```python
from build123d import *


with BuildPart() as part:
    # Sketch1 → Revolve1 (revolve)
    with BuildSketch(Plane(origin=(0, 0, 0), x_dir=(0, 0, -1), z_dir=(1, 0, 0))):
        with BuildLine():
            Line((0.388232597, 1.5), (6.712787917, 1.5))
            ThreePointArc((6.712787917, 1.5), (6.400595054, 2.031506006), (6, 2.5))
            ThreePointArc((6, 2.5), (3.550510257, 3.5), (1.101020514, 2.5))
            ThreePointArc((1.101020514, 2.5), (0.700425461, 2.031506006), (0.388232597, 1.5))
        make_face()
        with BuildLine():
            Line((0, 1.5), (0.388232597, 1.5))
            ThreePointArc((0.388232597, 1.5), (0.700425461, 2.031506006), (1.101020514, 2.5))
            Line((1.101020514, 2.5), (0, 2.5))
            Line((0, 2.5), (0, 1.5))
        make_face()
        with BuildLine():
            Line((6.712787917, 1.5), (14, 1.5))
            Line((14, 1.5), (14, 3))
            Line((14, 3), (12, 3))
            Line((12, 3), (12, 2.5))
            Line((12, 2.5), (6, 2.5))
            ThreePointArc((6, 2.5), (6.400595054, 2.031506006), (6.712787917, 1.5))
        make_face()
    revolve(axis=Axis((0, 0, 0), (0, 0, -1)))


solid = part.part
```
For this review, take the finished solid that the model builds, in its own axes (mm). A direction names the side the tool comes from. Coordinates: 2 decimals unless noted, no trailing zeros. Order: outer loops, then holes, each group sorted by start corner. A loop starts at its lowest first (then second) coordinate and runs counter-clockwise, first axis right, second up. Notation, with made-up numbers: (60, 66) -> (73, 66) arc R23 cw to (73, 100) -> close; hole circle Ø2 at (73, -12). An arc over 180 degrees is marked (long way). Use CSV: the item, a comma, the result in double quotes. Start each with the question number.
Item 1: Draft analysis for pull direction Z (two halves, no side actions). For faces 4 (the face through (0, 2, 0)), 5 (the face through (-2.44, -0.54, -8.96)), 6 (the face through (-2.44, -0.54, -0.54)), state which applies: pulls with the +Z half, pulls with the -Z half, needs draft (parallel to the pull), parting line crosses it, or undercut.
Item 2: Insertion check: pin 1 (2 mm diameter, centred on y = 2, z = -5, fed in from -X); pin 2 (4 mm diameter, centred on x = 0, z = -4.5, fed in from -Y); pin 3 (1 mm diameter, centred on y = -0.5, z = -10, fed in from -X); pin 4 (1.5 mm diameter, centred on y = 1.5, z = -9.5, fed in from -X). Each pin has a flat end and moves straight along its axis. Give the tip position at first contact, or say it passes through.
Item 3: Wall thickness on probe 1 along X at (y, z) = (0, -3.5); probe 2 along X at (y, z) = (0, -7.25); probe 3 along Z at (x, y) = (1.25, 2.5): over which ranges is each line inside the solid? List them lowest first.
Item 4: For faces 1 (the face through (-1.3, -1.3, -14)), 2 (the face through (0, -3, -13)), 3 (the face through (2, -2, -12)), list the 3-axis set-ups (+Z, -Z, +X, -X, +Y, -Y) from which the entire face can be reached by the end or side of a thin tool; tool diameter is ignored.
Item 5: We need section C-C, the plane z = -9.75. Give the boundary of the cut face in (x, y), then the cut area to 3 significant figures.
Item 6: We need section A-A, the plane y = 0. Give the boundary of the cut face in (x, z).
Item 7: We need section D-D, the plane x = -1.75. Give the boundary of the cut face in (y, z).
Derived:
1,face 4,"pulls with the +Z half"
1,face 5,"undercut"
1,face 6,"needs draft"
2,pin 1,"stops at x = -3.18"
2,pin 2,"stops at y = -3.5"
2,pin 3,"stops at x = -2.5"
2,pin 4,"stops at x = -2.38"
3,probe 1,"x = -3.5 to -1.5, 1.5 to 3.5"
3,probe 2,"x = -2.5 to -1.5, 1.5 to 2.5"
3,probe 3,"z = -14 to -12, -5.66 to -1.44"
4,face 1,"-Z, +X, -X, +Y, -Y"
4,face 2,"-Z"
4,face 3,"none"
5,outline,"circle Ø5 at (0, 0); hole circle Ø3 at (0, 0)"
5,area,"12.6 mm^2"
6,outline,"(-3, -14) -> (-1.5, -14) -> (-1.5, 0) -> (-2.5, 0) -> (-2.5, -1.1) arc R3.5 ccw to (-2.5, -6) -> (-2.5, -12) -> (-3, -12) -> close; (1.5, -14) -> (3, -14) -> (3, -12) -> (2.5, -12) -> (2.5, -6) arc R3.5 ccw to (2.5, -1.1) -> (2.5, 0) -> (1.5, 0) -> close"
7,outline,"(-2.44, -14) -> (2.44, -14) -> (2.44, -12) -> (1.79, -12) -> (1.79, -6) arc R3.03 ccw to (1.79, -1.1) -> (1.79, 0) -> (-1.79, 0) -> (-1.79, -1.1) arc R3.03 ccw to (-1.79, -6) -> (-1.79, -12) -> (-2.44, -12) -> close"
